Check sheet for the modelled part. Datum: model origin and axes. Units: mm. Face numbers are marked on the shaded views. A direction names the side the tool comes from. Round coordinates to 2 decimals unless told otherwise and drop trailing zeros. Order: outer loops, then holes, each group sorted by start corner. A loop starts at its lowest first (then second) coordinate and runs counter-clockwise, first axis right, second up.
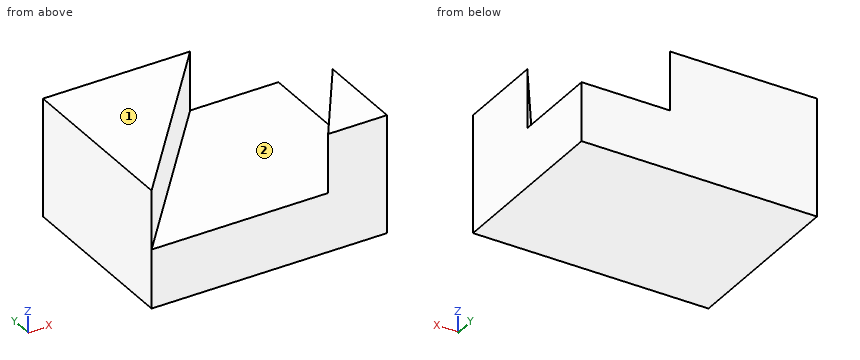
```python
from build123d import *

# Parameters (mm, degrees)
F0_W     = 101.6
F0_H     = 76.2
F1_DEPTH = 25.4
F3_DEPTH = 25.4
F5_DEPTH = 25.4


with BuildPart() as f1:
    # F0 (on Top) → F1 (new body)
    with BuildSketch(Plane.XY):
        with Locations((-2.955392, -5.993164)):
            Rectangle(F0_W, F0_H)
    extrude(amount=F1_DEPTH)

    # F2 (on face) → F3 (join)
    with BuildSketch(Plane.XY.offset(25.4)):
        Polygon((47.844608, -5.993164), (22.444608, -44.093164), (47.844608, -44.093164), align=None)
    extrude(amount=F3_DEPTH)

    # F4 (on face) → F5 (join)
    with BuildSketch(Plane.XY.offset(25.4)):
        Polygon((-53.755392, 32.106836), (-53.755392, -44.093164), (9.744608, 32.106836), align=None)
    extrude(amount=F5_DEPTH)


solid = f1.part
```
Item 1: Sectioned sample at C-C (x = 20). Record the cut outline in (y, z), and give its area (3 significant figures).
Answer:
outline: (-44.09, 0) - (32.11, 0) - (32.11, 25.4) - (-44.09, 25.4) - close
area: 1,940 mm2
Item 2: Sectioned sample at D-D (y = -38). Record the cut outline in (x, z).
Answer:
outline: (-53.76, 0) - (47.84, 0) - (47.84, 50.8) - (26.51, 50.8) - (26.51, 25.4) - (-48.68, 25.4) - (-48.68, 50.8) - (-53.76, 50.8) - close
Item 3: Sectioned sample at B-B (y = -15). Record the cut outline in (x, z), and give its area (3 significant figures).
Answer:
outline: (-53.76, 0) - (47.84, 0) - (47.84, 50.8) - (41.84, 50.8) - (41.84, 25.4) - (-29.51, 25.4) - (-29.51, 50.8) - (-53.76, 50.8) - close
area: 3,350 mm2
Item 4: Scan lines: line 1 along Z through (x, y) = (10.5, 3); line 2 along X through (y, z) = (9, 38); line 3 along X through (y, z) = (21, 42). Record each from-to range of solid material in increasing order.
Answer:
line 1: z = 0 to 25.4
line 2: x = -53.76 to -9.51
line 3: x = -53.76 to 0.49
Item 5: Access from +Z, -Z, +X, -X, +Y, -Y to the whole of each face (thin tool, end or side, straight path). Record for the marked faces 1 and 2.
Answer:
face 1: +Z, +X, -X, +Y, -Y
face 2: +Z
Item 6: Sectioned sample at A-A (z = 48). Record the cut outline in (x, y).
Answer:
outline: (-53.76, -44.09) - (9.74, 32.11) - (-53.76, 32.11) - close; (22.44, -44.09) - (47.84, -44.09) - (47.84, -5.99) - close
Item 7: Go/stop test with flat-tipped pins: P1, Ø12, axis at x = -4, y = -13, coming from the -Z side; P2, Ø23, axis at x = 16, y = 5, coming from the +Z side; P3, Ø10, axis at x = 8.5, z = 44, coming from the -Y side. Record where each tip stops, or that it passes through.
Answer:
P1: stops at z = 0
P2: stops at z = 25.4
P3: stops at y = 24.61
